```python
from build123d import *

# Parameters (mm, degrees)
SKETCH_W                 = 406.4
SKETCH_H                 = 406.4
SKETCH_W_2               = 304.8
SKETCH_H_2               = 304.8
PAD_DEPTH                = 1.5875
CLONE002_ROLL_ANGLE      = 90
CLONE002_PLACEMENT_ANGLE = 90
CLONE001_PLACEMENT_ANGLE = -90
CLONE003_PITCH_ANGLE     = -90
CLONE003_PLACEMENT_ANGLE = -90


with BuildPart() as left_frame:
    # Sketch → Pad (new body, symmetric)
    with BuildSketch(Plane.YZ):
        with Locations((203.2, 203.2)):
            Rectangle(SKETCH_W, SKETCH_H)
        with Locations((203.2, 203.2)):
            Rectangle(SKETCH_W_2, SKETCH_H_2, mode=Mode.SUBTRACT)
    extrude(amount=PAD_DEPTH, both=True)


with BuildPart() as back_frame:
    # Clone002 base: copy of Left Frame
    add(left_frame.part)


with BuildPart() as back_frame_1:
    # Clone002 roll: moved
    add(back_frame.part.rotate(Axis((0, 0, 0), (1, 0, 0)), CLONE002_ROLL_ANGLE))


with BuildPart() as back_frame_2:
    # Clone002 placement: moved
    add(back_frame_1.part.moved(Location((1.5875, 407.987, 0))).rotate(Axis((1.5875, 407.987, 0), (0, 0, 1)), CLONE002_PLACEMENT_ANGLE))


with BuildPart() as front_frame:
    # Clone001 base: copy of Left Frame
    add(left_frame.part)


with BuildPart() as front_frame_1:
    # Clone001 placement: moved
    add(front_frame.part.moved(Location((1.5875, -1.5875, 0))).rotate(Axis((1.5875, -1.5875, 0), (0, 0, 1)), CLONE001_PLACEMENT_ANGLE))


with BuildPart() as right_frame:
    # Clone base: copy of Left Frame
    add(left_frame.part)


with BuildPart() as right_frame_1:
    # Clone placement: moved
    add(right_frame.part.moved(Location((409.575, 0, 0))))


with BuildPart() as bottom_frame:
    # Clone003 base: copy of Left Frame
    add(left_frame.part)


with BuildPart() as bottom_frame_1:
    # Clone003 pitch: moved
    add(bottom_frame.part.rotate(Axis((0, 0, 0), (0, 1, 0)), CLONE003_PITCH_ANGLE))


with BuildPart() as bottom_frame_2:
    # Clone003 placement: moved
    add(bottom_frame_1.part.moved(Location((1.5875, 0, 0))).rotate(Axis((1.5875, 0, 0), (0, 0, 1)), CLONE003_PLACEMENT_ANGLE))


with BuildPart() as top_frame:
    # Clone004 base: copy of Bottom frame
    add(bottom_frame_2.part)


with BuildPart() as top_frame_1:
    # Clone004 placement: moved
    add(top_frame.part.moved(Location((0, 0, 406.4))))


with BuildPart() as frame:
    # Fusion005 base: copy of Bottom frame
    add(bottom_frame_2.part)

    # Fusion005: union Back Frame, Front Frame, Right Frame, Left Frame, Top Frame
    add(back_frame_2.part)
    add(front_frame_1.part)
    add(right_frame_1.part)
    add(left_frame.part)
    add(top_frame_1.part)


solid = frame.part
```
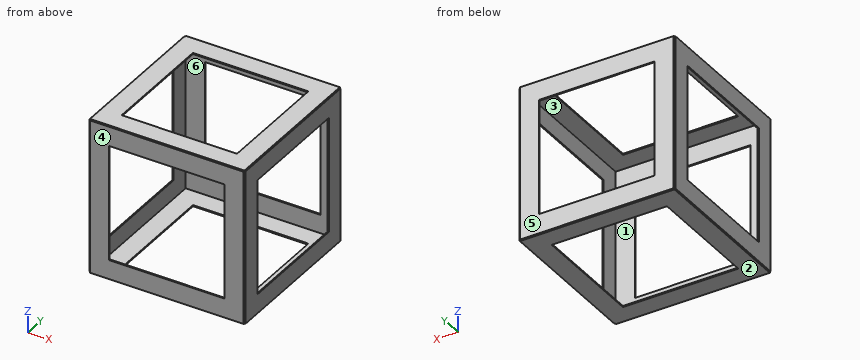
Read the model definition and answer for the solid it produces. Units are mm, in the model's axes. Face numbers are marked on the shaded views. A direction names the side the tool comes from. Give positions to 0.01 mm unless a question says otherwise; leave off trailing zeros. Write each loop counter-clockwise with the first axis right and the second up, starting at its lowest first coordinate (ties: lowest second). Pieces come first, ordered by that corner, then holes. Notation, with made-up numbers: (36, 47) -> (74, 47) arc R25 cw to (74, 76) -> close; hole circle Ø6 at (-30.5, 73). An arc over 180 degrees is marked (long way). Answer in a Markdown table with one row per item.
1) Section A-A on y = 158 is taken. Count the separate pieces of the cut face and the enclosed holes in it, plus the area to 3 significant figures.
Results list:
| item | result |
|---|---|
| separate pieces | 4 |
| enclosed holes | 0 |
| area | 1,290 mm^2 |
2) Section D-D on y = 24.5 is taken. Give the vertices of the cut face in (x, z).
Results list:
| item | result |
|---|---|
| outline | (-1.59, 0) -> (1.59, 0) -> (1.59, -1.59) -> (407.99, -1.59) -> (407.99, 0) -> (411.16, 0) -> (411.16, 406.4) -> (407.99, 406.4) -> (407.99, 407.99) -> (1.59, 407.99) -> (1.59, 406.4) -> (-1.59, 406.4) -> close; hole (1.59, 1.59) -> (407.99, 1.59) -> (407.99, 404.81) -> (1.59, 404.81) -> close |
3) A tool of negligible diameter and unlimited length cuts with its end or side. For the marked faces 5 and 6, from which of +Z, -Z, +X, -X, +Y, -Y can it reach the whole face along a straight path? Write none if from no direction.
Results list:
| item | result |
|---|---|
| face 5 | +Z, -Z, +X, -X, +Y |
| face 6 | none |
4) Straight lines are drawn through the part: line 1 (Z direction, x = 239, y = 50.5); line 2 (X direction, y = 217.5, z = 16); line 3 (Y direction, x = 136.5, z = 27.5) (1 decimal). For each, find the intervals that lie inside material, in ascending order. Write a range as [from, to].
Results list:
| item | result |
|---|---|
| line 1 | [-1.59, 1.59], [404.81, 407.99] |
| line 2 | [-1.59, 1.59], [407.99, 411.16] |
| line 3 | [-3.2, 0], [406.4, 409.6] |
5) Determine the mould class of the marked faces 1, 2, 3 and 4 for opening direction Z: released by +Z, released by -Z, zero draft, split by the parting line, or undercut.
Results list:
| item | result |
|---|---|
| face 1 | undercut |
| face 2 | released by -Z |
| face 3 | undercut |
| face 4 | zero draft |
6) Each of these flat-tipped pins is pushed along its axis until it touches: pin 1 Ø1.6 at (x, y) = (211, -2) entering from +Z; pin 2 Ø3.5 at (x, z) = (410, 218.5) entering from -Y; pin 3 Ø2.5 at (x, z) = (0, 279.5) entering from +Y. Where does it stop, or does it pass through?
Results list:
| item | result |
|---|---|
| pin 1 | z = 406.4 |
| pin 2 | y = 0 |
| pin 3 | y = 406.4 |
